CAD build for the part. Positions are in the model's coordinates, mm. A direction names the side the tool comes from. Round coordinates to 2 decimals unless told otherwise and drop trailing zeros. Loops run counter-clockwise (first coordinate to the right, second up) from the corner with the lowest first, then second, coordinate; pieces in that order, holes last.
Autodesk Inventor part; units mm, degrees
ref_plane "YZ Plane" through (0, 0, 0) normal (1, 0, 0) x (0, 1, 0)
ref_plane "XZ Plane" through (0, 0, 0) normal (0, 1, 0) x (-1, 0, 0)
ref_plane "XY Plane" through (0, 0, 0) normal (0, 0, 1) x (1, 0, 0)
sketch "Sketch23" plane through (0, 0, 0) normal (0, 1, 0) x (-1, 0, 0)
  line L0 (0, -7) -> (0, 42)
  line L1 (7, 0) -> (-42, 0)
  line L2 (0, 0) -> (-35, 0)
  line L3 (-35, 0) -> (-35, 35)
  line L4 (-35, 35) -> (0, 35)
  line L5 (0, 35) -> (0, 0)
  line L6 (0, 0) -> (-35, 35) construction
  point P0 (0, 0)
  dimension "d213" = 35
  dimension "d214" = 35
extrude "Extrusion14" add sketch "Sketch23" along normal blind 3
sketch "Sketch24" plane through (0, 3, 0) normal (0, 1, 0) x (1, 0, 0)
  line L0 (35, 0) -> (0, 0)
  line L1 (0, 0) -> (0, -35)
  line L2 (0, -35) -> (35, -35)
  line L3 (35, -35) -> (35, 0)
  line L4 (-41.7276, 41.7276) -> (35, -35) construction
  line L5 (-35.3553, 21.2132) -> (-21.2132, 35.3553)
  line L6 (-21.2132, 35.3553) -> (14.1421, 0)
  line L7 (35, 0) -> (0, 0)
  line L8 (0, -14.1421) -> (-35.3553, 21.2132)
  line L9 (-23.915, -23.915) -> (42.6519, 42.6519) construction
  dimension "d217" = 45
  dimension "d218" = 20
  dimension "d219" = 40
extrude "Extrusion15" add sketch "Sketch24" against normal blind 3 contours L0 L1 L8 L5 L6
sketch "Sketch36" plane through (0, 3, 0) normal (0, 1, 0) x (1, 0, 0)
  line L0 (-35.3553, 21.2132) -> (0, -14.1421)
  line L1 (14.1421, 0) -> (-21.2132, 35.3553)
  line L2 (-21.2132, 35.3553) -> (-35.3553, 21.2132)
  line L3 (-49.4264, 0) -> (49.0711, 0)
  line L4 (0, 49.4264) -> (0, -49.0711)
  line L5 (35, 0) -> (14.1421, 0)
  line L6 (0, -14.1421) -> (0, -35)
  line L7 (35, -35) -> (35, 0)
  line L8 (0, -35) -> (35, -35)
  line L9 (-30.4046, 30.4046) -> (24.5711, -24.5711) construction
  line L10 (14.1421, 0) -> (-21.2132, 35.3553)
  point P0 (0, 0)
  point P1 (0, -32)
  point P2 (32, 0)
  point P3 (-21.2132, 21.2132)
  dimension "d343" = 10
  dimension "d344" = 10
hole "Hole17" at (-21.2132, 3, -21.2132) direction (0, -1, 0) diameter 11 end through all
fillet "Fillet15" radius 10 2 edges at (-35.3553, 1.5, -21.2132) (-21.2132, 1.5, -35.3553)
fillet "Fillet18" radius 20 2 edges at (14.1421, 1.5, 0) (0, 1.5, 14.1421)
sketch "Sketch41" plane through (0, 3, 0) normal (0, 1, 0) x (1, 0, 0)
  line L0 (35, 0) -> (22.4264, 0)
  arc A0 (8.2843, 5.8579) -> (22.4264, 0) centre (22.4264, 20) ccw
  line L1 (8.2843, 5.8579) -> (-14.1421, 28.2843)
  arc A1 (-14.1421, 28.2843) -> (-28.2843, 14.1421) centre (-21.2132, 21.2132) ccw
  line L2 (-28.2843, 14.1421) -> (-5.8579, -8.2843)
  arc A2 (0, -22.4264) -> (-5.8579, -8.2843) centre (-20, -22.4264) ccw
  line L3 (0, -22.4264) -> (0, -35)
  line L4 (0, -35) -> (35, -35)
  line L5 (35, -35) -> (35, 0)
  circle A3 centre (-21.2132, 21.2132) radius 5.5
  line L6 (-42.9041, 42.9041) -> (81.0287, -81.0287) construction
  line L7 (8.2843, 5.8579) -> (-14.1421, 28.2843)
  line L8 (1.4985, 43.9249) -> (-47.6457, -5.2193) construction
  point P0 (0, 0)
  point P1 (0, 0)
  dimension "d365" = 30
hole "Hole20" at (0, 3, 0) direction (0, -1, 0) diameter 4 end through all
sketch "Sketch42" plane through (0, 3, 0) normal (0, 1, 0) x (1, 0, 0)
  circle A0 centre (0, 0) radius 2
  circle A1 centre (-21.2132, 21.2132) radius 5.5
  arc A2 (-14.1421, 28.2843) -> (-28.2843, 14.1421) centre (-21.2132, 21.2132) ccw
  line L0 (-28.2843, 14.1421) -> (-5.8579, -8.2843)
  arc A3 (0, -22.4264) -> (-5.8579, -8.2843) centre (-20, -22.4264) ccw
  line L1 (0, -22.4264) -> (0, -35)
  line L2 (0, -35) -> (35, -35)
  line L3 (35, -35) -> (35, 0)
  line L4 (35, 0) -> (22.4264, 0)
  arc A4 (8.2843, 5.8579) -> (22.4264, 0) centre (22.4264, 20) ccw
  line L5 (8.2843, 5.8579) -> (-14.1421, 28.2843)
  line L6 (35, -35) -> (15, -35)
  line L7 (15, -35) -> (15, -15)
  line L8 (15, -15) -> (35, -15)
  line L9 (35, -15) -> (35, -35)
  line L10 (35, -35) -> (35, 0)
  line L11 (0, -35) -> (35, -35)
  point P0 (0, 0)
  dimension "d423" = 15
  dimension "d424" = 15
extrude "Extrusion20" cut sketch "Sketch42" against normal blind 3 contours L3 L2 L7 L8
sketch "Sketch46" plane through (0, 3, 0) normal (0, 1, 0) x (1, 0, 0)
  line L0 (35, 0) -> (22.4264, 0)
  line L1 (0, -22.4264) -> (0, -35)
  line L2 (35, -15) -> (35, 0)
  line L3 (0, -35) -> (15, -35)
  point P0 (0, 0)
  point P1 (27, -5)
  point P2 (5, -27)
  dimension "d403" = 5
  dimension "d405" = 5
  dimension "d425" = 8
  dimension "d426" = 8
hole "Hole23" at (27, 3, 5) at (5, 3, 27) direction (0, -1, 0) diameter 4 end through all
fillet "Fillet22" radius 6 1 edges at (15, 1.5, 15)
properties part number "quarter_upper"
Item 1: Cut at B-B (y = 0.65). State how many separate pieces and enclosed holes the cut face has, plus the area to 3 significant figures.
Verdict:
separate pieces: 1
enclosed holes: 4
area: 1,570 mm2
Item 2: Mould opens along Z. For faces 6 (the cylindrical face through (14.874, 1.479, -1.481)), 7 (the cylindrical face through (4.399, 1.479, 28.908)), 8 (the flat face through (35, 1, 7)) say: released by +Z, released by -Z, zero draft, split by the parting line, or undercut.
Verdict:
face 6: released by -Z
face 7: undercut
face 8: zero draft
Item 3: Cut at A-A (z = 26). List the corners of the cut face in (x, y).
Verdict:
outline: (0, 0) - (3.27, 0) - (3.27, 3) - (0, 3) - close; (6.73, 0) - (15, 0) - (15, 3) - (6.73, 3) - close
Item 4: Cut at C-C (x = 5). List the corners of the cut face in (y, z).
Verdict:
outline: (0, -9.14) - (3, -9.14) - (3, 25) - (0, 25) - close; (0, 29) - (3, 29) - (3, 35) - (0, 35) - close
Item 5: Cut at D-D (x = 13). List the corners of the cut face in (y, z), plus the area to 3 significant figures.
Verdict:
outline: (0, -2.36) - (3, -2.36) - (3, 35) - (0, 35) - close
area: 112 mm2
Item 6: Wall check: L1, parallel to X at y = 1.6, z = 27; L2, parallel to X at y = 0.85, z = 5; L3, parallel to X at y = 2.45, z = -3. Give the ranges that are in metal, low to high.
Verdict:
L1: x = 0 to 3, 7 to 15
L2: x = -9.14 to 25, 29 to 35
L3: x = -17.14 to 11.89
Item 7: Flat gauge pins, fed straight in: P1, Ø1.5, axis at x = 25, y = 2, coming from the +Z side; P2, Ø0.9, axis at y = 1, z = 31.5, coming from the -X side; P3, Ø1.5, axis at x = 30.5, y = 1.5, coming from the -Z side. Where does each tip first touch, or does it go through?
Verdict:
P1: stops at z = 15
P2: stops at x = 0
P3: stops at z = 0
Item 8: 3-axis set-ups, long thin cutter, end or side, ignore diameter. For faces 1 (the flat face through (0, 1, 29)), 2 (the flat face through (15, 2, 28)), 3 (the flat face through (29, 1, 0)), 4 (the flat face through (2, 0, 2)), 5 (the cylindrical face through (-31.213, 1.479, -21.103)): which of +Z, -Z, +X, -X, +Y, -Y reach the whole face in a straight line?
Verdict:
face 1: +Z, -X, +Y, -Y
face 2: +Z, +X, +Y, -Y
face 3: -Z, +X, +Y, -Y
face 4: +Z, -Z, +X, -X, -Y
face 5: -X, +Y, -Y
